Read the model definition and answer for the solid it produces. Units are mm, in the model's axes. Face numbers are marked on the shaded views. A direction names the side the tool comes from. Round coordinates to 2 decimals unless told otherwise and drop trailing zeros. Write each loop counter-clockwise with the first axis right and the second up, starting at its lowest first coordinate (ties: lowest second). Pieces come first, ordered by that corner, then holes. Notation, with made-up numbers: (-26.5, -12) -> (12.5, -12) arc R29 cw to (12.5, 16) -> close; hole circle Ø11 at (70, -13). An arc over 180 degrees is marked (long way). Return JSON: item names as keys, results as strings.
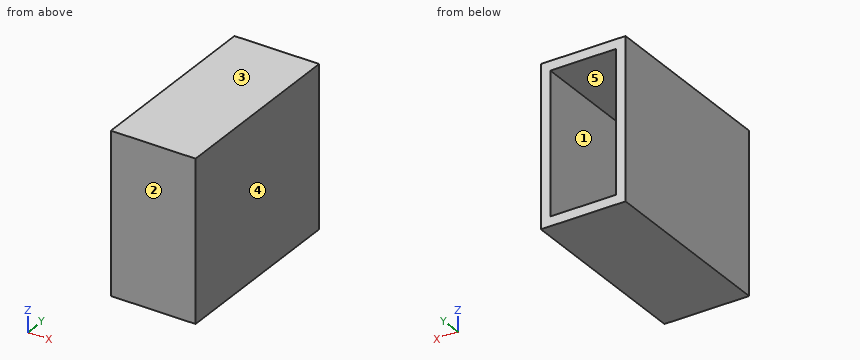
from build123d import *

# Parameters (mm, degrees)
SKETCH1_W           = 45
SKETCH1_H           = 85
BOSS_EXTRUDE1_DEPTH = 100
SHELL1_T            = -5
SKETCH2_W           = 3
SKETCH2_H           = 10
BOSS_EXTRUDE2_DEPTH = 15
SKETCH4_W           = 20
SKETCH4_H           = 2.5
BOSS_EXTRUDE3_DEPTH = 1
SKETCH5_W           = 15.809094042
SKETCH5_H           = 2
BOSS_EXTRUDE4_DEPTH = 1
SKETCH6_W           = 10
SKETCH6_H           = 2.5
BOSS_EXTRUDE5_DEPTH = 1
SKETCH9_W           = 10.477527882
SKETCH9_H           = 6.322646136
CUT_EXTRUDE1_DEPTH  = 9


with BuildPart() as part:
    # Sketch1 → Boss-Extrude1 (new body)
    with BuildSketch(Plane(origin=(0, 0, 0), x_dir=(1, 0, 0), z_dir=(0, 1, 0))):
        Rectangle(SKETCH1_W, SKETCH1_H)
    extrude(amount=BOSS_EXTRUDE1_DEPTH)

    # Shell1
    shell1_openings = [part.faces().sort_by_distance(p)[0] for p in [
        (0, 100, 0),
    ]]
    offset(amount=SHELL1_T, openings=shell1_openings, kind=Kind.INTERSECTION)

    # Sketch2 → Boss-Extrude2 (add)
    with BuildSketch(Plane(origin=(0, 5, 0), x_dir=(1, 0, 0), z_dir=(0, 1, 0))):
        with BuildLine():
            Line((-13.25, -29), (-13.25, -24))
            Line((-13.25, -24), (-16.25, -24))
            Line((-16.25, -24), (-16.25, -32))
            Line((-16.25, -32), (1.75, -32))
            Line((1.75, -32), (1.75, -16.155494421))
            ThreePointArc((1.75, -16.155494421), (0.251072202, -16.248060277), (-1.25, -16.201851746))
            Line((-1.25, -16.201851746), (-1.25, -29))
            Line((-1.25, -29), (-13.25, -29))
        make_face()
        with Locations((-14.75, -19)):
            Rectangle(SKETCH2_W, SKETCH2_H)
        with BuildLine():
            Line((-16.25, -14), (-13.25, -14))
            Line((-13.25, -14), (-13.25, -9.407443861))
            ThreePointArc((-13.25, -9.407443861), (-15.481844205, -4.937104415), (-16.25, 0))
            Line((-16.25, 0), (-16.25, -14))
        make_face()
        with BuildLine():
            Line((-4.205809483, 15.696294677), (-3.429352348, 12.798517198))
            ThreePointArc((-3.429352348, 12.798517198), (0, 13.25), (3.429352348, 12.798517198))
            Line((3.429352348, 12.798517198), (4.205809483, 15.696294677))
            ThreePointArc((4.205809483, 15.696294677), (0, 16.25), (-4.205809483, 15.696294677))
        make_face()
        with BuildLine():
            ThreePointArc((-16.25, 0), (-15.481844205, -4.937104415), (-13.25, -9.407443861))
            Line((-13.25, -9.407443861), (-13.25, 0))
            Line((-13.25, 0), (-16.25, 0))
        make_face()
        with BuildLine():
            Line((-1.25, -13.190905958), (-1.25, -16.201851746))
            ThreePointArc((-1.25, -16.201851746), (0.251072202, -16.248060277), (1.75, -16.155494421))
            Line((1.75, -16.155494421), (1.75, -13.133925537))
            ThreePointArc((1.75, -13.133925537), (0.251618147, -13.247610664), (-1.25, -13.190905958))
        make_face()
    extrude(amount=BOSS_EXTRUDE2_DEPTH)

    # Sketch4 → Boss-Extrude3 (add)
    with BuildSketch(Plane(origin=(-13.25, 0, 0), x_dir=(0, 0, -1), z_dir=(1, 0, 0))):
        with Locations((-19, 18.75)):
            Rectangle(SKETCH4_W, SKETCH4_H)
    extrude(amount=BOSS_EXTRUDE3_DEPTH)

    # Sketch5 → Boss-Extrude4 (add)
    with BuildSketch(Plane.ZY.offset(1.25)):
        with Locations((21.095452979, 19)):
            Rectangle(SKETCH5_W, SKETCH5_H)
    extrude(amount=BOSS_EXTRUDE4_DEPTH)

    # Sketch6 → Boss-Extrude5 (add)
    with BuildSketch(Plane(origin=(0, 0, 29), x_dir=(-1, 0, 0), z_dir=(0, 0, -1))):
        with Locations((7.25, 18.75)):
            Rectangle(SKETCH6_W, SKETCH6_H)
    extrude(amount=BOSS_EXTRUDE5_DEPTH)

    # Sketch9 → Cut-Extrude1 (cut)
    with BuildSketch(Plane(origin=(0, 20, 0), x_dir=(1, 0, 0), z_dir=(0, 1, 0))):
        with Locations((0.163497959, 14.216347227)):
            Rectangle(SKETCH9_W, SKETCH9_H)
    extrude(amount=-CUT_EXTRUDE1_DEPTH, mode=Mode.SUBTRACT)


solid = part.part
Item 1: For a pull along Z with two mould halves and no side action, classify the marked faces 1, 2 and 3 as released by +Z, released by -Z, zero draft, split by the parting line, or undercut.
Worked answers:
{"face 1": "undercut", "face 2": "zero draft", "face 3": "released by +Z"}
Item 2: Section A-A (y = 9.5) is taken. Give the vertices of the cut face in (x, z).
Worked answers:
{"outline": "(-22.5, -42.5) -> (22.5, -42.5) -> (22.5, 42.5) -> (-22.5, 42.5) -> close; (-16.25, 0) -> (-13.25, 0) -> (-13.25, 29) -> (-1.25, 29) -> (-1.25, 13.19) arc R13.25 cw to (1.75, 13.13) -> (1.75, 32) -> (-16.25, 32) -> close; (-4.21, -15.7) arc R16.25 ccw to (4.21, -15.7) -> (3.43, -12.8) arc R13.25 cw to (-3.43, -12.8) -> close; hole (-17.5, -37.5) -> (17.5, -37.5) -> (17.5, 37.5) -> (-17.5, 37.5) -> close"}
Item 3: A flat-ended cylindrical pin translates along its axis: pin 1 (8 mm diameter, centred on x = -17.5, z = 24.5, fed in from -Y). Find the tip coordinate at first contact, or state that the pin passes through.
Worked answers:
{"pin 1": "stops at y = 0"}
Item 4: Section B-B (y = 34) is taken. Give the vertices of the cut face in (x, z).
Worked answers:
{"outline": "(-22.5, -42.5) -> (22.5, -42.5) -> (22.5, 42.5) -> (-22.5, 42.5) -> close; hole (-17.5, -37.5) -> (17.5, -37.5) -> (17.5, 37.5) -> (-17.5, 37.5) -> close"}
Item 5: Section C-C (z = -9) is taken. Give the vertices of the cut face in (x, y).
Worked answers:
{"outline": "(-22.5, 0) -> (22.5, 0) -> (22.5, 100) -> (17.5, 100) -> (17.5, 5) -> (-17.5, 5) -> (-17.5, 100) -> (-22.5, 100) -> close"}
Item 6: A tool of negligible diameter and unlimited length cuts with its end or side. For the marked faces 4 and 5, from which of +Z, -Z, +X, -X, +Y, -Y can it reach the whole face along a straight path? Write none if from no direction.
Worked answers:
{"face 4": "+Z, -Z, +X, +Y, -Y", "face 5": "+Y"}
Item 7: Section D-D (x = -10) is taken. Give the vertices of the cut face in (y, z), then the cut area to 3 significant figures.
Worked answers:
{"outline": "(0, -42.5) -> (100, -42.5) -> (100, -37.5) -> (5, -37.5) -> (5, 29) -> (17.5, 29) -> (17.5, 28) -> (20, 28) -> (20, 32) -> (5, 32) -> (5, 37.5) -> (100, 37.5) -> (100, 42.5) -> (0, 42.5) -> close", "area": "1,420 mm2"}
Item 8: Straight lines are drawn through the part: L1, parallel to X at y = 10.5, z = 10; L2, parallel to Z at x = -11, y = 5.5; L3, parallel to X at y = 60, z = 31. For each, find the intervals that lie inside material, in ascending order. Write a range as [from, to].
Worked answers:
{"L1": "x = [-22.5, -17.5], [-16.25, -13.25], [17.5, 22.5]", "L2": "z = [-42.5, -37.5], [29, 32], [37.5, 42.5]", "L3": "x = [-22.5, -17.5], [17.5, 22.5]"}
